Here's how the part is built. I have some questions about the finished solid (model axes, mm). A direction names the side the tool comes from. Give positions to 0.01 mm unless a question says otherwise; leave off trailing zeros. Order: outer loops, then holes, each group sorted by start corner. A loop starts at its lowest first (then second) coordinate and runs counter-clockwise, first axis right, second up. Notation, with made-up numbers: (-26.75, -40) - (-0.75, -40) arc R27 cw to (-0.75, -23) - close; hole circle Ø5 at (-6.5, 15.5). An arc over 180 degrees is marked (long way). One line per question, with ' | ' between items.
from build123d import *

# Parameters (mm, degrees)
SKETCH_1_R               = 1.6
EXTRUDE_1_DEPTH          = 2.5
EXTRUDE_2_DEPTH          = 7
EXTRUDE_2_DEPTH_BACK     = 7
SKETCH_4_R               = 25
CUT_EXTRUDE_3_DEPTH      = 29.313247783
CUT_EXTRUDE_4_DEPTH      = 10
CUT_EXTRUDE_4_DEPTH_BACK = 10
SKETCH_7_R               = 9


with BuildPart() as part:
    # Sketch 1 → Extrude 1 (new body)
    with BuildSketch(Plane(origin=(0, 0, 0), x_dir=(1, 0, 0), z_dir=(0, 1, 0))):
        with BuildLine():
            Line((16.235294118, -4.941176471), (5.647058824, -10.588235294))
            ThreePointArc((5.647058824, -10.588235294), (0, -12), (-5.647058824, -10.588235294))
            Line((-5.647058824, -10.588235294), (-16.235294118, -4.941176471))
            ThreePointArc((-16.235294118, -4.941176471), (-19.2, 0), (-16.235294118, 4.941176471))
            Line((-16.235294118, 4.941176471), (-5.647058824, 10.588235294))
            ThreePointArc((-5.647058824, 10.588235294), (0, 12), (5.647058824, 10.588235294))
            Line((5.647058824, 10.588235294), (16.235294118, 4.941176471))
            ThreePointArc((16.235294118, 4.941176471), (19.2, 0), (16.235294118, -4.941176471))
        make_face()
        with Locations(Location((-13.6, 0, 0), (0, 0, 270))):
            Circle(SKETCH_1_R, mode=Mode.SUBTRACT)
        with Locations(Location((13.6, 0, 0), (0, 0, 270))):
            Circle(SKETCH_1_R, mode=Mode.SUBTRACT)
    extrude(amount=-EXTRUDE_1_DEPTH)

    # Sketch 2 → Extrude 2 (add, two sides: drawn at the far end of the back side and taken through both)
    with BuildSketch(Plane(origin=(0, 0, 0), x_dir=(0, 0, -1), z_dir=(1, 0, 0)).offset(-EXTRUDE_2_DEPTH_BACK)):
        Polygon((12, 0), (-12, 0), (-10, 5), (-10, 17), (10, 17), (10, 5), align=None)
    extrude(amount=EXTRUDE_2_DEPTH + EXTRUDE_2_DEPTH_BACK)

    # Sketch 4 → Cut-Extrude 3 (cut, through all)
    with BuildSketch(Plane(origin=(0, 0, 0), x_dir=(1, 0, 0), z_dir=(0, 1, 0))):
        Circle(SKETCH_4_R)
        with BuildLine():
            Line((5.647058824, -10.588235294), (7, -9.866666667))
            Line((7, -9.866666667), (16.235294118, -4.941176471))
            ThreePointArc((16.235294118, -4.941176471), (19.2, 0), (16.235294118, 4.941176471))
            Line((16.235294118, 4.941176471), (7, 9.866666667))
            Line((7, 9.866666667), (5.647058824, 10.588235294))
            ThreePointArc((5.647058824, 10.588235294), (2.9104275, 11.641710002), (0, 12))
            ThreePointArc((0, 12), (-2.9104275, 11.641710002), (-5.647058824, 10.588235294))
            Line((-5.647058824, 10.588235294), (-7, 9.866666667))
            Line((-7, 9.866666667), (-16.235294118, 4.941176471))
            ThreePointArc((-16.235294118, 4.941176471), (-19.2, 0), (-16.235294118, -4.941176471))
            Line((-16.235294118, -4.941176471), (-7, -9.866666667))
            Line((-7, -9.866666667), (-5.647058824, -10.588235294))
            ThreePointArc((-5.647058824, -10.588235294), (-2.9104275, -11.641710002), (0, -12))
            ThreePointArc((0, -12), (2.9104275, -11.641710002), (5.647058824, -10.588235294))
        make_face(mode=Mode.SUBTRACT)
    extrude(amount=CUT_EXTRUDE_3_DEPTH, mode=Mode.SUBTRACT)

    # Sketch 7 → Cut-Extrude 4 (cut, two sides: drawn at the far end of the back side and taken through both)
    with BuildSketch(Plane(origin=(0, 0, 0), x_dir=(0, 0, -1), z_dir=(1, 0, 0)).offset(-CUT_EXTRUDE_4_DEPTH_BACK)):
        with Locations((0, 17)):
            Circle(SKETCH_7_R)
    extrude(amount=CUT_EXTRUDE_4_DEPTH + CUT_EXTRUDE_4_DEPTH_BACK, mode=Mode.SUBTRACT)


solid = part.part
1) On a 3-axis mill with a long thin cutter (end or side, diameter ignored), from which of +Z, -Z, +X, -X, +Y, -Y can I reach the whole of each face in a straight line? I mean faces 4 (the face through (0, 11, 10)), 5 (the face through (-7, 5, 0)), 6 (the face through (11.8, 0, -0.1)). Say none if no direction works.
Model answer:
face 4: +Z, +X, -X, +Y | face 5: +Z, -Z, -X, +Y | face 6: +Z, -Z, +X, +Y
2) I'm going to push flat-ended pins straight in: P1, Ø8.5, axis at y = 5, z = 4.5, coming from the +X side; P2, Ø13.5, axis at x = -15.5, z = -4, coming from the +Y side; P3, Ø6, axis at y = 3.5, z = 1, coming from the -X side. Where does each tip first touch, or does it pass through?
Model answer:
P1: stops at x = 7 | P2: stops at y = 0 | P3: stops at x = -7
3) I want a section at B-B (x = 13.6). List the corners of the cut face in (y, z) for me, plus the area to 3 significant figures.
Model answer:
outline: (-2.5, -6.35) - (0, -6.35) - (0, -1.6) - (-2.5, -1.6) - close; (-2.5, 1.6) - (0, 1.6) - (0, 6.35) - (-2.5, 6.35) - close | area: 23.7 mm2
4) I want a section at A-A (y = 11.25). List the corners of the cut face in (x, z) for me, plus the area to 3 significant figures.
Model answer:
outline: (-7, -9.87) - (-6.75, -10) - (6.75, -10) - (7, -9.87) - (7, -6.92) - (-7, -6.92) - close; (-7, 6.92) - (7, 6.92) - (7, 9.87) - (6.75, 10) - (-6.75, 10) - (-7, 9.87) - close | area: 86.1 mm2
5) I want a section at C-C (z = -6.75). List the corners of the cut face in (x, y) for me.
Model answer:
outline: (-12.84, -2.5) - (12.84, -2.5) - (12.84, 0) - (7, 0) - (7, 11.05) - (-7, 11.05) - (-7, 0) - (-12.84, 0) - close
6) Please list where these lines run through material, in increasing order: L1, parallel to X at y = -1.4, z = 0; L2, parallel to X at y = 3.5, z = -4.25; L3, parallel to Y at x = -9.5, z = 0.5.
Model answer:
L1: x = -19.2 to -15.2, -12 to 12, 15.2 to 19.2 | L2: x = -7 to 7 | L3: y = -2.5 to 0
7) Thinking about a two-plate mould opening in Z: for faces 1 (the face through (-0.1, 3, 10.8)), 2 (the face through (0, 8, 0)), 3 (the face through (0, 11, -10)), which applies, +Z half, -Z half, draft (parallel to the pull), parting line (faces both ways), or undercut?
Model answer:
face 1: +Z half | face 2: undercut | face 3: -Z half
8) I want a section at D-D (x = -0.5). List the corners of the cut face in (y, z) for me.
Model answer:
outline: (-2.5, -11.99) - (0.03, -11.99) - (5, -10) - (17, -10) - (17, -9) arc R9 cw to (17, 9) - (17, 10) - (5, 10) - (0.03, 11.99) - (-2.5, 11.99) - close
